Work out the finished part from the listing and answer in its coordinate system (mm). A direction names the side the tool comes from. Round coordinates to 2 decimals unless told otherwise and drop trailing zeros. Order: outer loops, then holes, each group sorted by start corner. A loop starts at its lowest first (then second) coordinate and runs counter-clockwise, first axis right, second up. Notation, with made-up numbers: (-21.75, 16.5) - (-2.75, 16.5) arc R18 ccw to (-2.75, 50.5) - close; hole circle Ø6 at (-20, 87.5). An arc over 180 degrees is marked (long way). Answer in a Markdown table with one row per item.
Autodesk Inventor part; units mm, degrees
ref_plane "YZ Plane" through (0, 0, 0) normal (1, 0, 0) x (0, 1, 0)
ref_plane "XZ Plane" through (0, 0, 0) normal (0, 1, 0) x (-1, 0, 0)
ref_plane "XY Plane" through (0, 0, 0) normal (0, 0, 1) x (1, 0, 0)
sketch "Sketch1" plane through (0, 0, 0) normal (1, 0, 0) x (0, 1, 0)
  line L0 (-15.7, 12.7) -> (-12.7, 12.7)
  line L1 (-12.7, 12.7) -> (-12.7, -9.3)
  line L2 (-12.7, -9.3) -> (13.3, -9.3)
  line L3 (13.3, -9.3) -> (13.3, 13.1)
  line L4 (13.3, 13.1) -> (16.3, 13.1)
  line L5 (16.3, 13.1) -> (16.3, -12.3)
  line L6 (16.3, -12.3) -> (-15.7, -12.3)
  line L7 (-15.7, -12.3) -> (-15.7, 12.7)
  point P0 (0, 0)
  point P1 (0.3, 0.2)
  dimension "d0" = 3
  dimension "d1" = 3
  dimension "d2" = 25
  dimension "d3" = 32
  dimension "d4" = 16
  dimension "d5" = 12.5
  dimension "d6" = 3
  dimension "d44" = 22.4
  dimension "d45" = 16.3
  dimension "d46" = 13.1
extrude "Extrusion1" add sketch "Sketch1" along normal blind 482.6
sketch "Sketch3" plane through (0.7366, -15.7, 12.7) normal (0, -1, 0) x (1, 0, 0)
  line L0 (0, 0) -> (14.6558, -25.4)
  line L1 (-0.7366, -25) -> (481.8634, -25)
  line L2 (466.471, -25.4) -> (481.1268, 0)
  line L3 (-0.7366, 0) -> (481.8634, 0)
  line L4 (7.3279, -12.7) -> (473.7989, -12.7) construction
  line L5 (14.4316, 0) -> (28.8566, -25) construction
  circle A0 centre (21.6441, -12.5) radius 4.7625
  line L6 (466.6952, 0) -> (452.2702, -25) construction
  circle A1 centre (459.4827, -12.5) radius 4.7625
  point P0 (-0.7366, -12.7)
  dimension "d18" = 12.5
  dimension "d19" = 9.525
  dimension "d20" = 12.5
  dimension "d21" = 9.525
hole "Access Hole" at (22.3807, -15.7, 0.2) at (460.2193, -15.7, 0.2) direction (0, 1, 0) diameter 9.525 depth 3 tip angle 118
sketch "Sketch4" plane through (0.7366, 16.3, 12.7) normal (0, 1, 0) x (1, 0, 0)
  circle A0 centre (21.6441, 12.5) radius 4.7625
  circle A1 centre (459.4827, 12.5) radius 4.7625
  circle A2 centre (21.6441, 12.5) radius 3.175
  circle A3 centre (459.4827, 12.5) radius 3.175
  point P0 (-0.7366, 12.7)
  dimension "d29" = 6.35
  dimension "d30" = 6.35
hole "Mounting Hole" at (22.3807, 16.3, 0.2) at (460.2193, 16.3, 0.2) direction (0, -1, 0) diameter 6.35 depth 3 tip angle 118
chamfer "Chamfer1" distance 25 angle 30 1 edges at (0, 0.3, -12.3) measured on face at (0, 4.6333, -11.3)
chamfer "Chamfer2" distance 25 angle 30 1 edges at (482.6, 0.3, -12.3) measured on face at (482.6, 4.6333, -11.3)
sketch "Sketch5" plane through (0, -15.7, 12.7) normal (0, -1, 0) x (1, 0, 0)
  circle A0 centre (22.3807, -12.5) radius 4.7625
  circle A1 centre (460.2193, -12.5) radius 4.7625
  line L0 (0, 0) -> (482.6, 0)
  line L1 (14.4338, -25) -> (468.1662, -25)
  line L2 (51.0807, 0) -> (51.0807, -25) construction
  line L3 (431.5193, 0) -> (431.5193, -25) construction
  circle A2 centre (431.5193, -9.5) radius 3.175
  circle A3 centre (51.0807, -9.5) radius 3.175
  point P0 (0, -12.7)
  dimension "d47" = 28.7
  dimension "d49" = 28.7
  dimension "d61" = 6.35
  dimension "d62" = 15.5
  dimension "d63" = 6.35
  dimension "d71" = 51.0807
hole "Hole4" at (51.0807, -15.7, 3.2) at (431.5193, -15.7, 3.2) direction (0, 1, 0) diameter 6.35 depth 3 tip angle 118
equation "\"d1\" = d0"
equation "\"d6\" = d0"
equation "\"d19\" = d21"
equation "\"d49\" = d47"
properties part number "19in c-channel-top"
1) The mould has two halves that part along X. Classify faces 3 (the face through (238, -12.7, 2)), 4 (the face through (464.87, -14.18, 1.23)), 5 (the face through (17.66, -14.18, 0.82)), 6 (the face through (13.13, 2.75, -10.04)): released by +X, released by -X, zero draft, split by the parting line, or undercut.
Filled in:
| item | result |
|---|---|
| face 3 | zero draft |
| face 4 | undercut |
| face 5 | undercut |
| face 6 | released by -X |
2) Each of these flat-tipped pins is pushed along its axis until it touches: pin 1 (2.5 mm diameter, centred on x = 294.5, y = -14.5, fed in from +Z); pin 2 (12 mm diameter, centred on y = 9.5, z = -9.5, fed in from +X); pin 3 (7.5 mm diameter, centred on x = 22.38, z = 0.2, fed in from -Y). Where does it stop, or does it pass through?
Filled in:
| item | result |
|---|---|
| pin 1 | stops at z = 12.7 |
| pin 2 | stops at x = 472.46 |
| pin 3 | stops at y = 13.3 |
3) Find section B-B, the plane y = -1.5. Give the vertices of the cut face in (x, z).
Filled in:
| item | result |
|---|---|
| outline | (12.7, -9.3) - (14.43, -12.3) - (468.17, -12.3) - (469.9, -9.3) - close |
4) Which of the six approach directions +Z, -Z, +X, -X, +Y, -Y give full straight-line access (tool end or side, diameter ignored) to faces 1 (the face through (238, 13.3, 2)), 2 (the face through (238, 16.3, 1))?
Filled in:
| item | result |
|---|---|
| face 1 | +Z, +X, -X |
| face 2 | +Z, -Z, +X, -X, +Y |
5) Find the intervals of material crossed by probe 1 along Y at (x, z) = (243.5, -0.25); probe 2 along Z at (x, y) = (147.5, -3); probe 3 along X at (y, z) = (-12.5, -10.5), in increasing order. Write a range as from..to.
Filled in:
| item | result |
|---|---|
| probe 1 | y = -15.7..-12.7, 13.3..16.3 |
| probe 2 | z = -12.3..-9.3 |
| probe 3 | x = 13.39..469.21 |
6) Find section A-A, the plane x = 186.5. Give the vertices of the cut face in (y, z).
Filled in:
| item | result |
|---|---|
| outline | (-15.7, -12.3) - (16.3, -12.3) - (16.3, 13.1) - (13.3, 13.1) - (13.3, -9.3) - (-12.7, -9.3) - (-12.7, 12.7) - (-15.7, 12.7) - close |
